Autodesk Inventor part; units mm, degrees
ref_plane "YZ Plane" through (0, 0, 0) normal (1, 0, 0) x (0, 1, 0)
ref_plane "XZ Plane" through (0, 0, 0) normal (0, 1, 0) x (-1, 0, 0)
ref_plane "XY Plane" through (0, 0, 0) normal (0, 0, 1) x (1, 0, 0)
sketch "Sketch1" plane through (0, 0, 0) normal (0, 0, 1) x (1, 0, 0)
  circle A0 centre (0, 0) radius 15
  circle A1 centre (0, 0) radius 8.5
  line L0 (0, 8.5) -> (0, -8.5)
  circle A2 centre (0, 0) radius 3.75
  line L1 (18, -15) -> (-18, -15)
  line L2 (-18, -15) -> (-18, 15)
  line L3 (-18, 15) -> (18, 15)
  line L4 (18, 15) -> (18, -15)
  point P0 (0, 15)
  point P1 (0, -15)
  dimension "d0" = 30
  dimension "d1" = 17
  dimension "d2" = 7.5
  dimension "d15" = 30
  dimension "d16" = 36
  dimension "d17" = 18
  dimension "d18" = 15
extrude "Extrusion1" add sketch "Sketch1" along normal blind 10 contours A0 | A1 L0 A2 | L0 A2 A1
hole "Hole1" at (0, 8.5, 0) at (0, -8.5, 0) direction (0, 0, 1) diameter 3 end through all
sketch "Sketch2" plane through (0, 0, 10) normal (0, 0, 1) x (1, 0, 0)
  circle A0 centre (0, 0) radius 13
  dimension "d12" = 26
extrude "Extrusion2" cut sketch "Sketch2" against normal blind 2
extrude "Extrusion3" add sketch "Sketch1" along normal blind 10 contours A0 L3 L4 L1 | A0 L1 L2 L3
sketch "Sketch4" plane through (-18, -15, 0) normal (-1, 0, 0) x (0, 0, 1)
  line L0 (5, 27) -> (5, 3)
  line L1 (0, 30) -> (0, 0)
  line L2 (0, 0) -> (10, 0)
  line L3 (0, 30) -> (10, 30)
  point P0 (0, 15)
  dimension "d21" = 5
  dimension "d22" = 24
  dimension "d23" = 3
  dimension "d24" = 3
hole "Hole2" at (-18, 12, 5) at (-18, -12, 5) direction (1, 0, 0) diameter 2.8 end through all
sketch "Sketch5" plane through (18, -15, 0) normal (1, 0, 0) x (0, 0, -1)
  circle A0 centre (-5, 27) radius 1.4
  line L0 (-5, 27) -> (-5, 3)
  line L1 (0, 5) -> (-8, 5)
  point P0 (0, 15)
  dimension "d32" = 24
hole "Hole3" at (18, 12, 5) at (18, -12, 5) direction (-1, 0, 0) diameter 2.8 depth 8
sketch "Sketch6" plane through (-18, -15, 0) normal (0, -1, 0) x (1, 0, 0)
  line L0 (3, 8.3) -> (6, 8.3)
  line L1 (6, 8.3) -> (6, 1.7)
  line L2 (6, 1.7) -> (3, 1.7)
  line L3 (3, 1.7) -> (3, 8.3)
  line L4 (0, 10) -> (36, 10)
  line L5 (0, 0) -> (0, 10)
  line L6 (33, 8.3) -> (30, 8.3)
  line L7 (30, 8.3) -> (30, 1.7)
  line L8 (30, 1.7) -> (33, 1.7)
  line L9 (33, 1.7) -> (33, 8.3)
  line L10 (36, 0) -> (36, 10)
  line L11 (0, 0) -> (36, 0)
  point P0 (18, 0)
  dimension "d40" = 6.6
  dimension "d41" = 3
  dimension "d42" = 1.7
  dimension "d43" = 3
  dimension "d44" = 3
  dimension "d45" = 3
  dimension "d46" = 6.6
  dimension "d47" = 1.7
extrude "Extrusion4" cut sketch "Sketch6" against normal blind 7 contours L0 L1 L2 L3 | L9 L8 L7 L6
sketch "Sketch7" plane through (-18, 15, 0) normal (0, 1, 0) x (1, 0, 0)
  line L0 (33, -8.3) -> (30, -8.3)
  line L1 (30, -8.3) -> (30, -1.7)
  line L2 (30, -1.7) -> (33, -1.7)
  line L3 (33, -1.7) -> (33, -8.3)
  line L4 (3, -8.3) -> (6, -8.3)
  line L5 (6, -8.3) -> (6, -1.7)
  line L6 (6, -1.7) -> (3, -1.7)
  line L7 (3, -1.7) -> (3, -8.3)
  line L8 (0, 0) -> (0, -10)
  line L9 (36, 0) -> (36, -10)
  line L10 (36, 0) -> (0, 0)
  point P0 (18, 0)
  dimension "d50" = 3
  dimension "d51" = 3
  dimension "d52" = 3
  dimension "d53" = 3
  dimension "d54" = 1.7
  dimension "d55" = 1.7
  dimension "d56" = 6.6
  dimension "d57" = 6.6
extrude "Extrusion5" cut sketch "Sketch7" against normal blind 7
sketch "Sketch8" plane through (0, 0, 0) normal (0, 0, -1) x (-1, 0, 0)
  circle A0 centre (0, -8.5) radius 1.5
  circle A1 centre (0, 8.5) radius 1.5
  circle A2 centre (0, -8.5) radius 1.5
  circle A3 centre (0, -8.5) radius 3
  circle A4 centre (0, 8.5) radius 1.5
  circle A5 centre (0, 8.5) radius 3
  point P0 (0, 0)
  dimension "d60" = 6
  dimension "d61" = 6
extrude "Extrusion6" cut sketch "Sketch8" against normal blind 4
properties part number "motorfogo" material "PC/ABS Plastic"
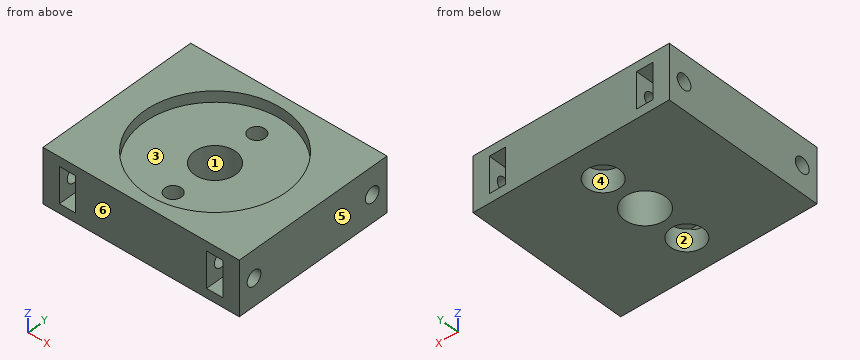
CAD build for the part. Positions are in the model's coordinates, mm. Face numbers are marked on the shaded views. A direction names the side the tool comes from. Give positions to 0.01 mm unless a question says otherwise; leave off trailing zeros. Write each loop counter-clockwise with the first axis right and the second up, starting at its lowest first coordinate (ties: lowest second). Pieces come first, ordered by that corner, then holes. Notation, with made-up numbers: M 75,4 L 113,4 A12 ccw 113,23 Z; hole C 18,44.25 d11. An arc over 180 degrees is marked long. Put each result on its own line as item: value. Start each with the question number.
(1) Band-saw the part on B-B, the plane y = 8.5. Write the cut outline in (x, z), and give its area (3 significant figures).
(2) Which spindle directions (+Z, -Z, +X, -X, +Y, -Y) get a long thin tool onto all of the face, cutting with end or side? Do the marked faces 1, 2 and 3. Say none if no direction does.
(3) Flat gauge pins, fed straight in: pin 1 Ø0.9 at (x, z) = (-13, 3.5) entering from +Y; pin 2 Ø8 at (x, y) = (-1, 2.5) entering from +Z. Where does each tip first touch, or does it go through?
(4) Probe L1, parallel to Y at x = 0, z = 2.5; L2, parallel to X at y = -8.5, z = 2.95; L3, parallel to Y at x = -17.15, z = 5. List the from-to ranges inside material, lowest first.
(5) Band-saw the part on A-A, the plane y = 0. Write the cut outline in (x, z).
(6) Mould opens along Y. For the marked faces 4, 5 and 6 say: +Y half, -Y half, draft (parallel to the pull), parting line (faces both ways), or undercut.
(7) Band-saw the part on D-D, the plane x = -5. Write the cut outline in (y, z).
(8) Band-saw the part on C-C, the plane z = 1. Write the cut outline in (x, y), and give its area (3 significant figures).
Response values:
1. outline: M -18,0 L -3,0 L -3,4 L -1.5,4 L -1.5,8 L -9.84,8 L -9.84,10 L -18,10 Z; M 1.5,4 L 3,4 L 3,0 L 18,0 L 18,10 L 9.84,10 L 9.84,8 L 1.5,8 Z; hole M -15,1.7 L -12,1.7 L -12,8.3 L -15,8.3 Z; hole M 12,1.7 L 15,1.7 L 15,8.3 L 12,8.3 Z
1. area: 245 mm2
2. face 1: +Z, -Z
2. face 2: -Z
2. face 3: +Z
3. pin 1: stops at y = 8
3. pin 2: stops at z = 8
4. L1: y = -15 to -11.5, -5.5 to -3.75, 3.75 to 5.5, 11.5 to 15
4. L2: x = -18 to -15, -12 to -3, 3 to 12, 15 to 18
4. L3: y = -15 to -13.4, -10.6 to 10.6, 13.4 to 15
5. outline: M -18,0 L -3.75,0 L -3.75,8 L -13,8 L -13,10 L -18,10 Z; M 3.75,0 L 18,0 L 18,10 L 13,10 L 13,8 L 3.75,8 Z
6. face 4: undercut
6. face 5: draft
6. face 6: -Y half
7. outline: M -15,0 L 15,0 L 15,10 L 12,10 L 12,8 L -12,8 L -12,10 L -15,10 Z; hole C -12,5 d2.8; hole C 12,5 d2.8
8. outline: M -18,-15 L 18,-15 L 18,15 L -18,15 Z; hole C 0,0 d7.5; hole C 0,-8.5 d6; hole C 0,8.5 d6
8. area: 979 mm2
